For this review, use the dimensioned drawing (mm, ordinates from the lowest corner) and the shaded views. Coordinates: 2 decimals unless noted, no trailing zeros. Write each loop counter-clockwise with the first axis right and the second up, starting at its lowest first coordinate (ties: lowest second). Pieces come first, ordered by that corner, then holes.
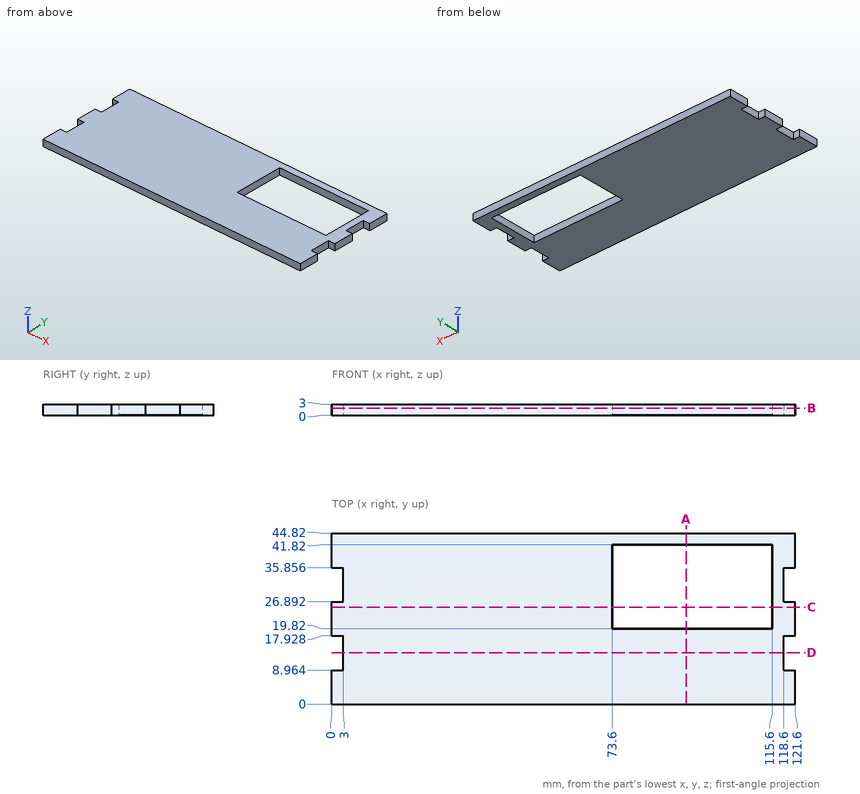
(1) Insertion check: pin 1 Ø0.9 at (y, z) = (12.5, 1) entering from +X; pin 2 Ø0.9 at (y, z) = (30.5, 2) entering from -X; pin 3 Ø0.9 at (x, z) = (91, 1.5) entering from -Y. Each pin has a flat end and moves straight along its axis. Give the tip position at first contact, or say it passes through.
(2) Consider section C-C (y = 25.5). Give the boundary of the cut face in (x, z).
(3) Consider section A-A (x = 93). Give the boundary of the cut face in (y, z), plus the area to 3 significant figures.
(4) Consider section B-B (z = 1.95). Give the boundary of the cut face in (x, y).
(5) Consider section D-D (y = 13.5). Give the boundary of the cut face in (x, z), plus the area to 3 significant figures.
(6) Wall thickness on line 1 (Y direction, x = 115, z = 0.3); line 2 (X direction, y = 30, z = 2.1); line 3 (X direction, y = 21, z = 2.25): over which ranges is each line inside the solid? List them lowest first.
Results:
1. pin 1: stops at x = 118.6
1. pin 2: stops at x = 3
1. pin 3: stops at y = 0
2. outline: (0, 0) - (73.6, 0) - (73.6, 3) - (0, 3) - close; (115.6, 0) - (121.6, 0) - (121.6, 3) - (115.6, 3) - close
3. outline: (0, 0) - (19.82, 0) - (19.82, 3) - (0, 3) - close; (41.82, 0) - (44.82, 0) - (44.82, 3) - (41.82, 3) - close
3. area: 68.5 mm2
4. outline: (0, 0) - (121.6, 0) - (121.6, 8.96) - (118.6, 8.96) - (118.6, 17.93) - (121.6, 17.93) - (121.6, 26.89) - (118.6, 26.89) - (118.6, 35.86) - (121.6, 35.86) - (121.6, 44.82) - (0, 44.82) - (0, 35.86) - (3, 35.86) - (3, 26.89) - (0, 26.89) - (0, 17.93) - (3, 17.93) - (3, 8.96) - (0, 8.96) - close; hole (73.6, 19.82) - (115.6, 19.82) - (115.6, 41.82) - (73.6, 41.82) - close
5. outline: (3, 0) - (118.6, 0) - (118.6, 3) - (3, 3) - close
5. area: 347 mm2
6. line 1: y = 0 to 19.82, 41.82 to 44.82
6. line 2: x = 3 to 73.6, 115.6 to 118.6
6. line 3: x = 0 to 73.6, 115.6 to 121.6
